Source: three-view drawing plus pictorial views. Frame: mm from the lowest corner of the part. A direction names the side the tool comes from. Give positions to 0.01 mm unless a question says otherwise; leave off trailing zeros. Loops run counter-clockwise (first coordinate to the right, second up) from the corner with the lowest first, then second, coordinate; pieces in that order, holes last. Notation, with made-up numbers: (15, 28.5) - (27, 28.5) arc R7 ccw to (27, 41.5) - close; hole circle Ø10 at (62.25, 75). An arc over 180 degrees is marked (long way). Answer as a JSON object with one key per item and string values.
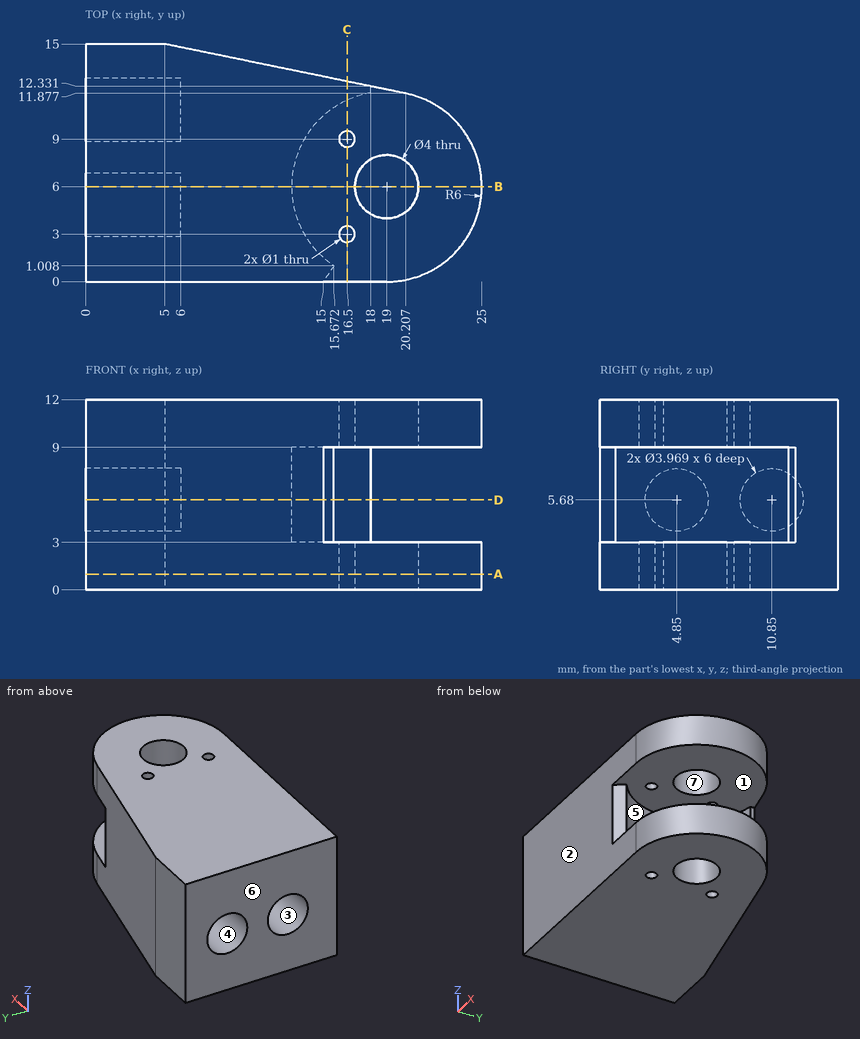
Item 1: Cut plane A-A (z = 1). Return loops of the section in (x, y), then the cut area to 3 significant figures.
Geometry check:
{"outline": "(0, 0) - (19, 0) arc R6 ccw to (20.21, 11.88) - (5, 15) - (0, 15) - close; hole circle Ø1 at (16.5, 3); hole circle Ø1 at (16.5, 9); hole circle Ø4 at (19, 6)", "area": "307 mm2"}
Item 2: Cut plane C-C (x = 16.5). Return loops of the section in (y, z) (1 decimal).
Geometry check:
{"outline": "(0, 0) - (2.5, 0) - (2.5, 3) - (0, 3) - close; (0, 9) - (2.5, 9) - (2.5, 12) - (0, 12) - close; (3.5, 0) - (8.5, 0) - (8.5, 3) - (3.5, 3) - close; (3.5, 9) - (8.5, 9) - (8.5, 12) - (3.5, 12) - close; (9.5, 0) - (12.6, 0) - (12.6, 12) - (9.5, 12) - (9.5, 9) - (11.5, 9) - (11.5, 3) - (9.5, 3) - close"}
Item 3: Material intervals for line 1 (Z direction, x = 17, y = 7.75); line 2 (Y direction, x = 16.5, z = 1.6); line 3 (Z direction, x = 1, y = 9.25) (1 decimal), sorted ascending. Write a range as [from, to].
Geometry check:
{"line 1": "z = [0, 3], [9, 12]", "line 2": "y = [0, 2.5], [3.5, 8.5], [9.5, 12.64]", "line 3": "z = [0, 4.5], [6.9, 12]"}
Item 4: Cut plane B-B (y = 6). Return loops of the section in (x, z).
Geometry check:
{"outline": "(0, 0) - (17, 0) - (17, 3) - (13, 3) - (13, 9) - (17, 9) - (17, 12) - (0, 12) - (0, 7.3) - (6, 7.3) - (6, 4.06) - (0, 4.06) - close; (21, 0) - (25, 0) - (25, 3) - (21, 3) - close; (21, 9) - (25, 9) - (25, 12) - (21, 12) - close"}
Item 5: Access query for the marked faces 1, 2 and 3. Directions: +Z, -Z, +X, -X, +Y, -Y. A direction counts if a zero-diameter tool reaches every point of the face in a straight line with its end or side. Return the directions, or none.
Geometry check:
{"face 1": "+X", "face 2": "+Z, -Z, +X, -X, -Y", "face 3": "-X"}
Item 6: Cut plane D-D (z = 5.68). Return loops of the section in (x, y) (1 decimal), then the cut area to 3 significant figures.
Geometry check:
{"outline": "(0, 0) - (15, 0) - (15.7, 1) arc R6 cw to (18, 11.9) - (18, 12.3) - (5, 15) - (0, 15) - (0, 12.8) - (6, 12.8) - (6, 8.9) - (0, 8.9) - (0, 6.8) - (6, 6.8) - (6, 2.9) - (0, 2.9) - close", "area": "159 mm2"}
Item 7: Mould query, pull axis X, two halves, no side actions, for the marked faces 4, 5, 6 and 7. Classes: released by +X, released by -X, zero draft, split by the parting line, or undercut.
Geometry check:
{"face 4": "zero draft", "face 5": "released by +X", "face 6": "released by -X", "face 7": "undercut"}
Item 8: Contact query for flat-ended pins moving along their axis: P1, Ø3.5, axis at x = 22, y = 7, coming from the -Z side; P2, Ø1.5, axis at x = 21, z = 2, coming from the +Y side; P3, Ø3, axis at y = 4.85, z = 5.68, coming from the -X side; P4, Ø6.5, axis at y = 10.85, z = 5.68, coming from the +X side. Output: stop coordinate, or through.
Geometry check:
{"P1": "stops at z = 0", "P2": "stops at y = 11.87", "P3": "stops at x = 6", "P4": "stops at x = 24.19"}
